The listing builds one solid part. Answer for the finished solid, in the listing's coordinates (mm). Give positions to 0.01 mm unless a question says otherwise; leave off trailing zeros. Loops run counter-clockwise (first coordinate to the right, second up) from the corner with the lowest first, then second, coordinate; pieces in that order, holes last. Notation, with made-up numbers: M 44.25,79.5 L 83.25,79.5 A19 cw 83.25,95.5 Z; hole C 22.25,5 d2. An arc over 180 degrees is marked long. Use one line per item in the form item = value. Start each with the question number.
1. Straight lines are drawn through the part: line 1 (X direction, y = 5.5, z = 46.5); line 2 (Z direction, x = -70.5, y = 0.75); line 3 (Z direction, x = 11, y = 4.25). For each, find the intervals that lie inside material, in ascending order. Write a range as from..to.
2. The part is cut by section A-A (x = 2). Write down the section's boundary in (y, z).
3. The part is cut by section B-B (y = 2.5). Give the number of separate pieces and of enclosed holes in the cut face, and give its area (3 significant figures).
4. This flat-tipped pin is pushed along its axis until it touches: pin 1 Ø1.9 at (x, z) = (45.04, 27.21) entering from -Y. Where does it stop, or does it pass through?
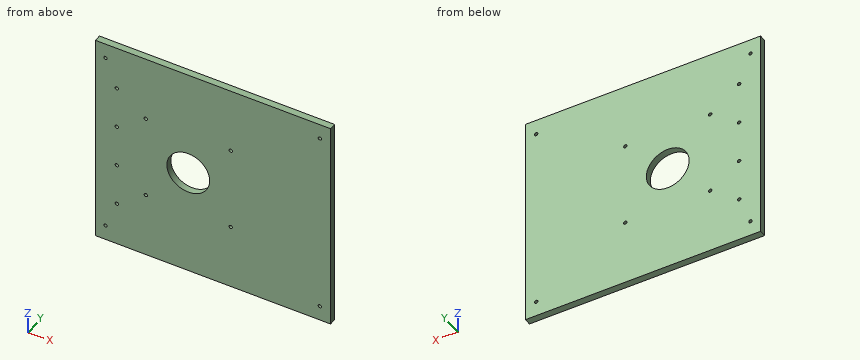
from build123d import *

# Parameters (mm, degrees)
SKETCH1_W           = 219.71
SKETCH1_H           = 203.2
BOSS_EXTRUDE1_DEPTH = 6.35
SKETCH2_R           = 1.5875
SKETCH2_R_2         = 20.000000005
CUT_EXTRUDE3_DEPTH  = 7.35


with BuildPart() as part:
    # Sketch1 → Boss-Extrude1 (new body)
    with BuildSketch(Plane(origin=(0, 0, 0), x_dir=(1, 0, 0), z_dir=(0, 1, 0))):
        with Locations((28.489079589, -66.894525566)):
            Rectangle(SKETCH1_W, SKETCH1_H)
    extrude(amount=BOSS_EXTRUDE1_DEPTH)

    # Sketch2 → Cut-Extrude3 (cut, through all)
    with BuildSketch(Plane(origin=(0, 6.35, 0), x_dir=(1, 0, 0), z_dir=(0, 1, 0))):
        with Locations((-61.365920533, -46.894525561)):
            Circle(SKETCH2_R)
        with Locations((128.298379589, -154.143525566)):
            Circle(SKETCH2_R)
        with Locations((128.298379589, 20.354474434)):
            Circle(SKETCH2_R)
        with Locations((-71.955220411, 20.354474434)):
            Circle(SKETCH2_R)
        with Locations((-71.955220411, -154.143525566)):
            Circle(SKETCH2_R)
        with Locations((-61.365920533, -6.894525551)):
            Circle(SKETCH2_R)
        with Locations((-61.365920533, -86.894525571)):
            Circle(SKETCH2_R)
        with Locations((-61.365920533, -126.894525327)):
            Circle(SKETCH2_R)
        with Locations((5.381145499, -66.894525566)):
            Circle(SKETCH2_R_2)
        with Locations((45.036895499, -106.582025566)):
            Circle(SKETCH2_R)
        with Locations((-34.306354501, -106.582025566)):
            Circle(SKETCH2_R)
        with Locations((-34.306354501, -27.207025566)):
            Circle(SKETCH2_R)
        with Locations((45.036895499, -27.207025566)):
            Circle(SKETCH2_R)
    extrude(amount=-CUT_EXTRUDE3_DEPTH, mode=Mode.SUBTRACT)


solid = part.part
Derived:
q1.line_1 = -81.37..-62.9, -59.83..138.34
q1.line_2 = -34.71..-20.99, -19.72..153.51, 154.78..168.49
q1.line_3 = -34.71..47.7, 86.09..168.49
q2.outline = M 0,-34.71 L 6.35,-34.71 L 6.35,47.18 L 0,47.18 Z; M 0,86.61 L 6.35,86.61 L 6.35,168.49 L 0,168.49 Z
q3.separate_pieces = 1
q3.enclosed_holes = 13
q3.area = 43,300 mm2
q4.pin_1 = through
